Work out the finished part from the listing and answer in its coordinate system (mm). Give positions to 0.01 mm unless a question says otherwise; leave off trailing zeros. Loops run counter-clockwise (first coordinate to the right, second up) from the corner with the lowest first, then second, coordinate; pieces in that order, holes last. Notation, with made-up numbers: (38.5, 45) -> (55.5, 45) arc R22 ccw to (55.5, 56) -> close; hole circle Ø11 at (4, 43). An arc over 180 degrees is marked (long way). Answer as CSV lines item,"result". Start each with the question number.
1. Find the intervals of material crossed by line 1 along X through (y, z) = (0.3, 1); line 2 along Z through (x, y) = (2, 0.4); line 3 along X through (y, z) = (0.85, 1.75), in increasing order.
2. Find section C-C, the plane y = 0.25. Give the vertices of the cut face in (x, z) (3 decimals).
3. Find section B-B, the plane x = 0.25. Give the vertices of the cut face in (y, z).
4. Find section A-A, the plane z = 0. Give the vertices of the cut face in (x, y), and give its area (3 significant figures).
5. Find section D-D, the plane x = -3.5. Give the vertices of the cut face in (y, z).
6. A flat-ended cylindrical pin translates along its axis: pin 1 Ø0.6 at (y, z) = (0.5, -4) entering from +X. Find the tip coordinate at first contact, or state that the pin passes through.
7. Determine the mould class of faces 1 (the face through (2, 1.25, 2)), 2 (the face through (0.125, 1, -3)), 3 (the face through (-0.125, 1, -3)) for opening direction X: +X half, -X half, draft (parallel to the pull), parting line (faces both ways), or undercut.
from build123d import *

# Parameters (mm, degrees)
SKETCH1_R               = 4.3
SKETCH1_R_2             = 2.6
BOSS_EXTRUDE1_DEPTH     = 1.25
SKETCH2_W               = 0.25
SKETCH2_H               = 4.3
CUT_EXTRUDE1_DEPTH      = 7.208260626
BODY_MOVE_COPY1_DEPTH   = 1.25
BODY_MOVE_COPY1_2_DEPTH = 1.25


# Read off the part's stored shape, not the designer's step: Body-Move/Copy1
with BuildPart() as part:
    # Sketch1 → Boss-Extrude1 (new body)
    with BuildSketch(Plane(origin=(0, 0, 0), x_dir=(1, 0, 0), z_dir=(0, 1, 0))):
        with Locations(Location((0, 0, 0), (0, 0, 270))):
            Circle(SKETCH1_R)
        with Locations(Location((0, 0, 0), (0, 0, 270))):
            Circle(SKETCH1_R_2, mode=Mode.SUBTRACT)
    extrude(amount=BOSS_EXTRUDE1_DEPTH)

    # Sketch2 → Cut-Extrude1 (cut, through all)
    with BuildSketch(Plane.XZ):
        with Locations((0, 2.15)):
            Rectangle(SKETCH2_W, SKETCH2_H)
    extrude(amount=-CUT_EXTRUDE1_DEPTH, mode=Mode.SUBTRACT)

    # Body-Move/Copy1 outline → Body-Move/Copy1 (cut)
    with BuildSketch(Plane(origin=(0, 0, 0), x_dir=(1, 0, 0), z_dir=(0, 1, 0))):
        with BuildLine():
            Line((0.125, 2.596993454), (0.125, 4.298182756))
            ThreePointArc((0.125, 4.298182756), (0, 4.3), (-0.125, 4.298182756))
            Line((-0.125, 4.298182756), (-0.125, 2.596993454))
            ThreePointArc((-0.125, 2.596993454), (0, 2.6), (0.125, 2.596993454))
        make_face()
    extrude(amount=BODY_MOVE_COPY1_DEPTH, mode=Mode.SUBTRACT)

    # Body-Move_Copy1 2 outline → Body-Move_Copy1 2 (add)
    with BuildSketch(Plane(origin=(0, 0, 0), x_dir=(1, 0, 0), z_dir=(0, 1, 0))):
        with BuildLine():
            ThreePointArc((-0.125, -4.298182756), (0, -4.3), (0.125, -4.298182756))
            Line((0.125, -4.298182756), (0.125, -2.596993454))
            ThreePointArc((0.125, -2.596993454), (0, -2.6), (-0.125, -2.596993454))
            Line((-0.125, -2.596993454), (-0.125, -4.298182756))
        make_face()
    extrude(amount=BODY_MOVE_COPY1_2_DEPTH)


solid = part.part
Resolved:
1,line 1,"x = -4.18 to -2.4, 2.4 to 4.18"
1,line 2,"z = -3.81 to -1.66, 1.66 to 3.81"
1,line 3,"x = -3.93 to -1.92, 1.92 to 3.93"
2,outline,"(-0.125, -4.298) -> (-0.125, -2.597) arc R2.6 cw (long way) to (0.125, -2.597) -> (0.125, -4.298) arc R4.3 ccw to (0.125, 4.298) arc R4.3 ccw to (-0.125, 4.298) arc R4.3 ccw to start"
3,outline,"(0, -4.29) -> (1.25, -4.29) -> (1.25, -2.59) -> (0, -2.59) -> close; (0, 2.59) -> (1.25, 2.59) -> (1.25, 4.29) -> (0, 4.29) -> close"
4,outline,"(-4.3, 0) -> (-2.6, 0) -> (-2.6, 1.25) -> (-4.3, 1.25) -> close; (2.6, 0) -> (4.3, 0) -> (4.3, 1.25) -> (2.6, 1.25) -> close"
4,area,"4.25 mm^2"
5,outline,"(0, -2.5) -> (1.25, -2.5) -> (1.25, 2.5) -> (0, 2.5) -> close"
6,pin 1,"stops at x = 2.19"
7,face 1,"draft"
7,face 2,"undercut"
7,face 3,"undercut"
